```python
from build123d import *

# Parameters (mm, degrees)
SKETCH_1_R      = 103.5
SKETCH_1_R_2    = 93.5
SKETCH_1_R_3    = 1.6
EXTRUDE_1_DEPTH = 3.5


with BuildPart() as part:
    # 草图1 → 凸台-拉伸1 (new body)
    with BuildSketch(Plane.XY):
        Circle(SKETCH_1_R)
        Circle(SKETCH_1_R_2, mode=Mode.SUBTRACT)
        with Locations((0, 98.5)):
            Circle(SKETCH_1_R_3, mode=Mode.SUBTRACT)
        with Locations((15.408794806, 97.287301549)):
            Circle(SKETCH_1_R_3, mode=Mode.SUBTRACT)
        with Locations((30.438173946, 93.679066855)):
            Circle(SKETCH_1_R_3, mode=Mode.SUBTRACT)
        with Locations((44.718064224, 87.764142633)):
            Circle(SKETCH_1_R_3, mode=Mode.SUBTRACT)
        with Locations((57.896847351, 79.688173946)):
            Circle(SKETCH_1_R_3, mode=Mode.SUBTRACT)
        with Locations((69.650017947, 69.650017947)):
            Circle(SKETCH_1_R_3, mode=Mode.SUBTRACT)
        with Locations((79.688173946, 57.896847351)):
            Circle(SKETCH_1_R_3, mode=Mode.SUBTRACT)
        with Locations((87.764142633, 44.718064224)):
            Circle(SKETCH_1_R_3, mode=Mode.SUBTRACT)
        with Locations((93.679066855, 30.438173946)):
            Circle(SKETCH_1_R_3, mode=Mode.SUBTRACT)
        with Locations((97.287301549, 15.408794806)):
            Circle(SKETCH_1_R_3, mode=Mode.SUBTRACT)
        with Locations((98.5, 0)):
            Circle(SKETCH_1_R_3, mode=Mode.SUBTRACT)
        with Locations((97.287301549, -15.408794806)):
            Circle(SKETCH_1_R_3, mode=Mode.SUBTRACT)
        with Locations((93.679066855, -30.438173946)):
            Circle(SKETCH_1_R_3, mode=Mode.SUBTRACT)
        with Locations((87.764142633, -44.718064224)):
            Circle(SKETCH_1_R_3, mode=Mode.SUBTRACT)
        with Locations((79.688173946, -57.896847351)):
            Circle(SKETCH_1_R_3, mode=Mode.SUBTRACT)
        with Locations((69.650017947, -69.650017947)):
            Circle(SKETCH_1_R_3, mode=Mode.SUBTRACT)
        with Locations((57.896847351, -79.688173946)):
            Circle(SKETCH_1_R_3, mode=Mode.SUBTRACT)
        with Locations((44.718064224, -87.764142633)):
            Circle(SKETCH_1_R_3, mode=Mode.SUBTRACT)
        with Locations((30.438173946, -93.679066855)):
            Circle(SKETCH_1_R_3, mode=Mode.SUBTRACT)
        with Locations((15.408794806, -97.287301549)):
            Circle(SKETCH_1_R_3, mode=Mode.SUBTRACT)
        with Locations((0, -98.5)):
            Circle(SKETCH_1_R_3, mode=Mode.SUBTRACT)
        with Locations((-15.408794806, -97.287301549)):
            Circle(SKETCH_1_R_3, mode=Mode.SUBTRACT)
        with Locations((-30.438173946, -93.679066855)):
            Circle(SKETCH_1_R_3, mode=Mode.SUBTRACT)
        with Locations((-44.718064224, -87.764142633)):
            Circle(SKETCH_1_R_3, mode=Mode.SUBTRACT)
        with Locations((-57.896847351, -79.688173946)):
            Circle(SKETCH_1_R_3, mode=Mode.SUBTRACT)
        with Locations((-69.650017947, -69.650017947)):
            Circle(SKETCH_1_R_3, mode=Mode.SUBTRACT)
        with Locations((-79.688173946, -57.896847351)):
            Circle(SKETCH_1_R_3, mode=Mode.SUBTRACT)
        with Locations((-87.764142633, -44.718064224)):
            Circle(SKETCH_1_R_3, mode=Mode.SUBTRACT)
        with Locations((-93.679066855, -30.438173946)):
            Circle(SKETCH_1_R_3, mode=Mode.SUBTRACT)
        with Locations((-97.287301549, -15.408794806)):
            Circle(SKETCH_1_R_3, mode=Mode.SUBTRACT)
        with Locations((-98.5, 0)):
            Circle(SKETCH_1_R_3, mode=Mode.SUBTRACT)
        with Locations((-97.287301549, 15.408794806)):
            Circle(SKETCH_1_R_3, mode=Mode.SUBTRACT)
        with Locations((-93.679066855, 30.438173946)):
            Circle(SKETCH_1_R_3, mode=Mode.SUBTRACT)
        with Locations((-87.764142633, 44.718064224)):
            Circle(SKETCH_1_R_3, mode=Mode.SUBTRACT)
        with Locations((-79.688173946, 57.896847351)):
            Circle(SKETCH_1_R_3, mode=Mode.SUBTRACT)
        with Locations((-69.650017947, 69.650017947)):
            Circle(SKETCH_1_R_3, mode=Mode.SUBTRACT)
        with Locations((-57.896847351, 79.688173946)):
            Circle(SKETCH_1_R_3, mode=Mode.SUBTRACT)
        with Locations((-44.718064224, 87.764142633)):
            Circle(SKETCH_1_R_3, mode=Mode.SUBTRACT)
        with Locations((-30.438173946, 93.679066855)):
            Circle(SKETCH_1_R_3, mode=Mode.SUBTRACT)
        with Locations((-15.408794806, 97.287301549)):
            Circle(SKETCH_1_R_3, mode=Mode.SUBTRACT)
    extrude(amount=EXTRUDE_1_DEPTH)


solid = part.part
```
The model under review builds one solid part; all positions refer to its coordinate system, in mm. Round coordinates to 2 decimals unless told otherwise and drop trailing zeros. Order: outer loops, then holes, each group sorted by start corner. A loop starts at its lowest first (then second) coordinate and runs counter-clockwise, first axis right, second up. Notation, with made-up numbers: (20, 15) -> (65, 15) arc R17 cw to (65, 28) -> close; hole circle Ø8 at (61.5, 81.5). An arc over 180 degrees is marked (long way). Use a Markdown table: item, result.
Q1. We need section B-B on x = 53. Write out the cut boundary in (y, z).
Values:
| item | result |
|---|---|
| outline | (-88.9, 0) -> (-77.03, 0) -> (-77.03, 3.5) -> (-88.9, 3.5) -> close; (77.03, 0) -> (88.9, 0) -> (88.9, 3.5) -> (77.03, 3.5) -> close |
Q2. Clearance check with flat-ended pins moving along their axes: P1, Ø2, axis at x = 80.5, z = 2.5, coming from the +Y side; P2, Ø3, axis at x = -93.68, y = 30.44, coming from the -Z side; P3, Ø1.5, axis at x = 43, z = 1, coming from the +Y side; P4, Ø1, axis at x = -36.5, z = 3, coming from the +Y side. State where each tip first meets the part, or that it passes through.
Values:
| item | result |
|---|---|
| P1 | stops at y = 66.27 |
| P2 | passes through |
| P3 | stops at y = 94.48 |
| P4 | stops at y = 97.04 |
Q3. We need section A-A on y = -9. Write out the cut boundary in (x, z), then the cut area to 3 significant figures.
Values:
| item | result |
|---|---|
| outline | (-103.11, 0) -> (-93.07, 0) -> (-93.07, 3.5) -> (-103.11, 3.5) -> close; (93.07, 0) -> (103.11, 0) -> (103.11, 3.5) -> (93.07, 3.5) -> close |
| area | 70.3 mm^2 |
Q4. We need section C-C on z = 2.1. State how many separate pieces and enclosed holes the cut face has, then the cut area to 3 significant figures.
Values:
| item | result |
|---|---|
| separate pieces | 1 |
| enclosed holes | 41 |
| area | 5,870 mm^2 |
Q5. For line 1 (Y direction, x = -30, z = 1.15); line 2 (X direction, y = 44, z = 2.8); line 3 (X direction, y = 58, z = 2.1), list the stretches that pass through material, from the lowest coordinate up.
Values:
| item | result |
|---|---|
| line 1 | y = -99.06 to -95.22, -92.14 to -88.56, 88.56 to 92.14, 95.22 to 99.06 |
| line 2 | x = -93.68 to -89.19, -86.33 to -82.5, 82.5 to 86.33, 89.19 to 93.68 |
| line 3 | x = -85.72 to -81.28, -78.09 to -73.34, 73.34 to 78.09, 81.28 to 85.72 |
Q6. Mouldability with a two-part tool opening along X and no side actions: class faces 1 (the cylindrical face through (98.72, 31.09, 1.73)), 2 (the cylindrical face through (50.265, 78.84, 1.726)), 3 (the flat face through (-77.1, -53.2, 0)) as +X half, -X half, draft (parallel to the pull), parting line (faces both ways), or undercut.
Values:
| item | result |
|---|---|
| face 1 | parting line |
| face 2 | undercut |
| face 3 | draft |
